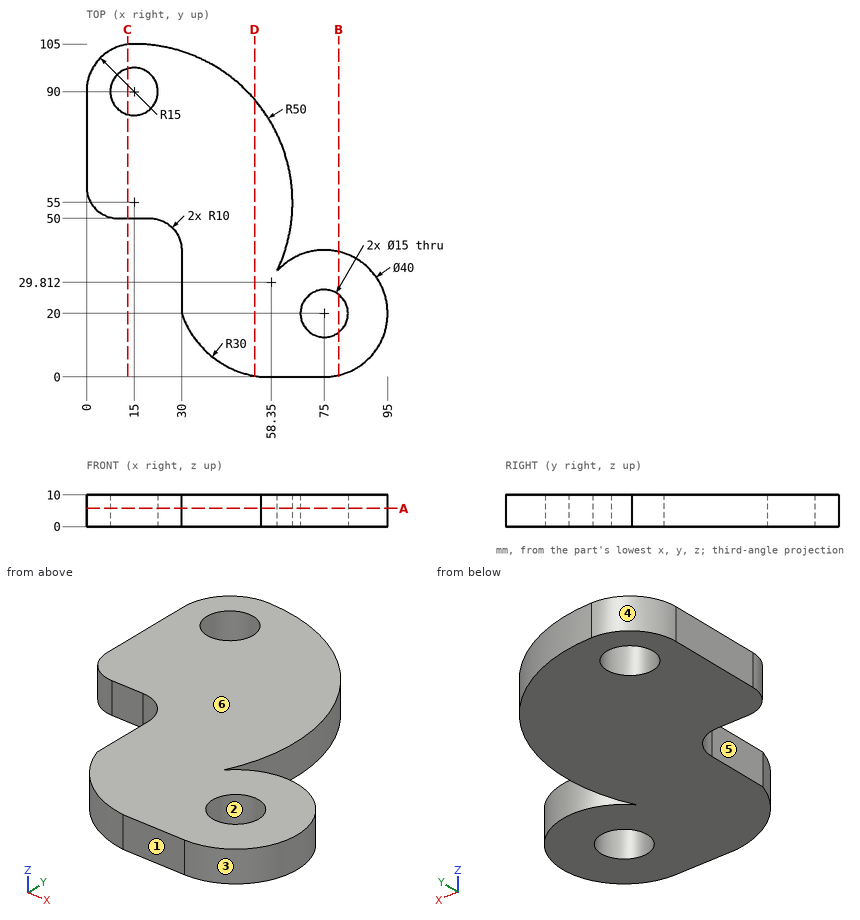
The drawing under review shows one solid part. Ordinate dimensions are in mm from its lowest x, y, z. A direction names the side the tool comes from. Round coordinates to 2 decimals unless told otherwise and drop trailing zeros. Write each loop counter-clockwise with the first axis right and the second up, starting at its lowest first coordinate (ties: lowest second). Pieces come first, ordered by that corner, then holes.
(1) We need section C-C on x = 13. Give the boundary of the cut face in (y, z), and give its area (3 significant figures).
(2) Wall thickness on L1, parallel to Y at x = 15, z = 4; L2, parallel to X at y = 87.5, z = 6.5 (1 decimal); L3, parallel to X at y = 83.5, z = 7 (1 decimal): over which ranges is each line inside the solid? List them lowest first.
(3) We need section D-D on x = 53. Give the boundary of the cut face in (y, z).
(4) Mouldability with a two-part tool opening along X and no side actions: class the marked faces 1, 2, 3 and 4 as +X half, -X half, draft (parallel to the pull), parting line (faces both ways), or undercut.
(5) Machinability: for the marked faces 5 and 6, which of the approach directions +Z, -Z, +X, -X, +Y, -Y give a long, thin tool a straight path to every point of the face, cutting with its end or side? Answer none if there is none.
(6) Insertion check: pin 1 (1.5 mm diameter, centred on x = 22, z = 2.5, fed in from +Y); pin 2 (13.5 mm diameter, centred on x = 15, y = 90, fed in from +Z); pin 3 (2 mm diameter, centred on y = 18.5, z = 3.5, fed in from +X); pin 4 (5 mm diameter, centred on y = 34, z = 2, fed in from +X). Each pin has a flat end and moves straight along its axis. Give the tip position at first contact, or say it passes through.
(7) We need section A-A on z = 5.75. Give the number of separate pieces and of enclosed holes in the cut face, and give its area (3 significant figures).
(8) We need section B-B on x = 79.5. Give the boundary of the cut face in (y, z), and give its area (3 significant figures).
Findings below:
1. outline: (50, 0) - (82.77, 0) - (82.77, 10) - (50, 10) - close; (97.23, 0) - (104.87, 0) - (104.87, 10) - (97.23, 10) - close
1. area: 404 mm2
2. L1: y = 50 to 82.5, 97.5 to 105
2. L2: x = 0 to 7.9, 22.1 to 53
2. L3: x = 0 to 11.3, 18.7 to 56.1
3. outline: (0.29, 0) - (87.5, 0) - (87.5, 10) - (0.29, 10) - close
4. face 1: draft
4. face 2: undercut
4. face 3: undercut
4. face 4: -X half
5. face 5: +Z, -Z, -X, -Y
5. face 6: +Z, +X, -X, +Y, -Y
6. pin 1: stops at y = 104.61
6. pin 2: passes through
6. pin 3: stops at x = 94.99
6. pin 4: stops at x = 91.36
7. separate pieces: 1
7. enclosed holes: 2
7. area: 5,230 mm2
8. outline: (0.51, 0) - (14, 0) - (14, 10) - (0.51, 10) - close; (26, 0) - (39.49, 0) - (39.49, 10) - (26, 10) - close
8. area: 270 mm2
